Input: part model. Units: mm. Frame: model coordinates. A direction names the side the tool comes from. Give positions to 0.01 mm unless a question says otherwise; leave off trailing zeros. Loops run counter-clockwise (first coordinate to the right, second up) from the corner with the lowest first, then second, coordinate; pieces in that order, holes last. Notation, with made-up numbers: (65, 86) -> (70, 86) arc R22 ccw to (70, 111) -> close; hole circle Ø9 at (80, -1). An arc over 180 degrees is marked (long way). One line per question, with ' | ' between items.
from build123d import *

# Parameters (mm, degrees)
SKETCH1_R           = 42.5
BOSS_EXTRUDE1_DEPTH = 10
SKETCH2_R           = 12.5
BOSS_EXTRUDE2_DEPTH = 10
SKETCH3_R           = 9
CUT_EXTRUDE1_DEPTH  = 20
SKETCH4_R           = 3.390899264
CUT_EXTRUDE2_DEPTH  = 10
CIRPATTERN1_COUNT   = 8


with BuildPart() as part:
    # Sketch1 → Boss-Extrude1 (new body)
    with BuildSketch(Plane.XY):
        Circle(SKETCH1_R)
    extrude(amount=BOSS_EXTRUDE1_DEPTH)

    # Sketch2 → Boss-Extrude2 (add)
    with BuildSketch(Plane.XY.offset(10)):
        Circle(SKETCH2_R)
    extrude(amount=BOSS_EXTRUDE2_DEPTH)

    # Sketch3 → Cut-Extrude1 (cut)
    with BuildSketch(Plane.XY.offset(20)):
        Circle(SKETCH3_R)
    extrude(amount=-CUT_EXTRUDE1_DEPTH, mode=Mode.SUBTRACT)

    # Sketch4 → Cut-Extrude2 (cut)
    with BuildSketch(Plane.XY.offset(10)):
        with Locations((0, 32.696600748)):
            Circle(SKETCH4_R)
    cut_extrude2 = extrude(amount=-CUT_EXTRUDE2_DEPTH, mode=Mode.SUBTRACT)

    # CirPattern1: Cut-Extrude2 ×8 about axis
    cirpattern1_axis = Axis((0, 0, 0), (0, 0, 1))
    for i in range(1, CIRPATTERN1_COUNT):
        add(cut_extrude2.rotate(cirpattern1_axis, i * 360 / CIRPATTERN1_COUNT), mode=Mode.SUBTRACT)


solid = part.part
1. Reachability of faces 1 (the flat face through (9, -9, 10)), 2 (the cylindrical face through (-19.99, 24.42, 5.07)) from +Z, -Z, +X, -X, +Y, -Y: full face, straight path, thin tool, end or side. Return the list, or none.
Determined:
face 1: +Z | face 2: +Z, -Z
2. Pin query (flat end, axial travel): P1, Ø10, axis at y = -33, z = 13, coming from the -X side; P2, Ø8, axis at y = -21, z = 5.5, coming from the +X side; P3, Ø2, axis at y = -10, z = 7.5, coming from the +X side; P4, Ø6, axis at x = 9.5, y = -13, coming from the -Z side. Return the tip coordinate at first contact, or that it passes through.
Determined:
P1: stops at x = -31.07 | P2: stops at x = 38.95 | P3: stops at x = 41.54 | P4: stops at z = 0
3. Ray query, line 1 along Y through (x, z) = (0, 7.75); line 2 along Y through (x, z) = (0, 14); line 3 along X through (y, z) = (0.5, 16.75). Return the intervals inside material, ascending. Write a range as from..to.
Determined:
line 1: y = -42.5..-36.09, -29.31..-9, 9..29.31, 36.09..42.5 | line 2: y = -12.5..-9, 9..12.5 | line 3: x = -12.49..-8.99, 8.99..12.49
4. Pull-direction query (Y, two-part tool) for faces 3 (the flat face through (-10, 1, 0)), 4 (the cylindrical face through (0.44, -36.06, 5.07)), 5 (the cylindrical face through (11.923, 3.755, 14.93)); classes: pulls with the +Y half, pulls with the -Y half, needs draft (parallel to the pull), parting line crosses it, or undercut.
Determined:
face 3: needs draft | face 4: undercut | face 5: parting line crosses it
5. Section query C-C (y = 24). Output: boundary loops of the cut face in (x, z), then the cut area to 3 significant figures.
Determined:
outline: (-35.07, 0) -> (-26.39, 0) -> (-26.39, 10) -> (-35.07, 10) -> close; (-19.85, 0) -> (19.85, 0) -> (19.85, 10) -> (-19.85, 10) -> close; (26.39, 0) -> (35.07, 0) -> (35.07, 10) -> (26.39, 10) -> close | area: 571 mm2
6. Section query D-D (z = 15). Output: boundary loops of the cut face in (x, y), then the cut area to 3 significant figures.
Determined:
outline: circle Ø25 at (0, 0); hole circle Ø18 at (0, 0) | area: 236 mm2
7. Section query A-A (y = 0). Output: boundary loops of the cut face in (x, z), then the cut area to 3 significant figures.
Determined:
outline: (-42.5, 0) -> (-36.09, 0) -> (-36.09, 10) -> (-42.5, 10) -> close; (-29.31, 0) -> (-9, 0) -> (-9, 20) -> (-12.5, 20) -> (-12.5, 10) -> (-29.31, 10) -> close; (9, 0) -> (29.31, 0) -> (29.31, 10) -> (12.5, 10) -> (12.5, 20) -> (9, 20) -> close; (36.09, 0) -> (42.5, 0) -> (42.5, 10) -> (36.09, 10) -> close | area: 604 mm2
